```python
from build123d import *

# Parameters (mm, degrees)
F0_W     = 825
F0_H     = 200
F1_DEPTH = 400
F2_T     = -1
F5_D     = 40
F7_D     = 30


# Not quite as in the source:
# - the program builds the solid bodies; features that only make, move or delete a surface that nothing else refers to are left out


with BuildPart() as f1:
    # F0 (on Top) → F1 (new body)
    with BuildSketch(Plane.XY):
        Rectangle(F0_W, F0_H)
    extrude(amount=F1_DEPTH)

    # F2
    f2_openings = [f1.faces().sort_by_distance(p)[0] for p in [
        (0, 0, 400),
    ]]
    offset(amount=F2_T, openings=f2_openings)

    # F5 (through all)
    with Locations(Plane.XY.offset(1)):
        with Locations((389.5, 77), (389.5, -77), (-389.5, 77), (-389.5, -77)):
            Hole(F5_D / 2)

    # F7 (through all)
    with Locations(Plane(origin=(-412.5, 0, 0), x_dir=(0, -1, 0), z_dir=(-1, 0, 0))):
        with Locations((0, 50)):
            Hole(F7_D / 2)


solid = f1.part
```
Could you check a few things on this model? Use its own coordinates, in mm. A direction names the side the tool comes from. Round coordinates to 2 decimals unless told otherwise and drop trailing zeros. Loops run counter-clockwise (first coordinate to the right, second up) from the corner with the lowest first, then second, coordinate; pieces in that order, holes last. Notation, with made-up numbers: (-36, 29.5) - (20, 29.5) arc R9 ccw to (20, 37.5) - close; hole circle Ø8 at (56, 10.5). An arc over 180 degrees is marked (long way). Answer in a Markdown table with one row per item. Add a question column.
(1) For faces 1 (the face through (371.025, 69.34, 0.493)), 2 (the face through (-6, 99, 198)), which set-ups out of +Z, -Z, +X, -X, +Y, -Y let a thin tool reach every point of the face, with its end or its side?
(2) I'm going to push a flat-ended pin straight in: pin 1 (1.5 mm diameter, centred on x = 19, y = -44.5, fed in from +Z). Where does the tip first touch, or does it pass through?
(3) I need wall thicknesses on line 1 along Y through (x, z) = (389.5, 0.5); line 2 along X through (y, z) = (-82.5, 353); line 3 along Z through (x, y) = (412.05, 0). Which ranges of each line are inside material? Lowest first, please.
(4) If we section it at D-D (x = -91.5): Please give me the cut outline in (y, z), plus the area to 3 significant figures.
(5) If we section it at C-C (z = 50): Please give me the cut outline in (x, y), plus the area to 3 significant figures.
(6) If we section it at B-B (x = -389.5): Please give me the cut outline in (y, z), plus the area to 3 significant figures.
(7) If we section it at A-A (y = 0): Please give me the cut outline in (x, z), plus the area to 3 significant figures.
(8) If we mould it in two halves opening along X, with no side actions, what happens to faces 3 (the face through (-6, 1, 1)), 4 (the face through (-412.5, -1, 197)), 5 (the face through (-411.993, -1.953, 64.872))? For each: pulls with the +X half, pulls with the -X half, needs draft (parallel to the pull), parting line crosses it, or undercut.
Model answer:
| question | item | result |
|---|---|---|
| 1 | face 1 | +Z, -Z |
| 1 | face 2 | +Z |
| 2 | pin 1 | stops at z = 1 |
| 3 | line 1 | y = -100 to -97, -57 to 57, 97 to 100 |
| 3 | line 2 | x = -412.5 to -411.5, 411.5 to 412.5 |
| 3 | line 3 | z = 0 to 35, 65 to 400 |
| 4 | outline | (-100, 0) - (100, 0) - (100, 400) - (99, 400) - (99, 1) - (-99, 1) - (-99, 400) - (-100, 400) - close |
| 4 | area | 998 mm² |
| 5 | outline | (-412.5, -100) - (412.5, -100) - (412.5, -15) - (411.5, -15) - (411.5, -99) - (-411.5, -99) - (-411.5, -15) - (-412.5, -15) - close; (-412.5, 15) - (-411.5, 15) - (-411.5, 99) - (411.5, 99) - (411.5, 15) - (412.5, 15) - (412.5, 100) - (-412.5, 100) - close |
| 5 | area | 1,990 mm² |
| 6 | outline | (-100, 0) - (-97, 0) - (-97, 1) - (-99, 1) - (-99, 400) - (-100, 400) - close; (-57, 0) - (57, 0) - (57, 1) - (-57, 1) - close; (97, 0) - (100, 0) - (100, 400) - (99, 400) - (99, 1) - (97, 1) - close |
| 6 | area | 918 mm² |
| 7 | outline | (-412.5, 0) - (412.5, 0) - (412.5, 35) - (411.5, 35) - (411.5, 1) - (-411.5, 1) - (-411.5, 35) - (-412.5, 35) - close; (-412.5, 65) - (-411.5, 65) - (-411.5, 400) - (-412.5, 400) - close; (411.5, 65) - (412.5, 65) - (412.5, 400) - (411.5, 400) - close |
| 7 | area | 1,560 mm² |
| 8 | face 3 | undercut |
| 8 | face 4 | pulls with the -X half |
| 8 | face 5 | needs draft |
